from build123d import *

# Parameters (mm, degrees)
SKETCH1_W           = 42
SKETCH1_H           = 42
SKETCH1_R           = 1.7
SKETCH1_R_2         = 11.5
BOSS_EXTRUDE1_DEPTH = 4
SKETCH2_W           = 55
SKETCH2_H           = 80
SKETCH2_R           = 4.05
SKETCH2_W_2         = 36
SKETCH2_H_2         = 29
BOSS_EXTRUDE2_DEPTH = 10
BOSS_EXTRUDE4_DEPTH = 30.5
SKETCH5_W           = 42
SKETCH5_H           = 26.825
BOSS_EXTRUDE5_DEPTH = 42
SKETCH6_R           = 1.7
CUT_EXTRUDE1_DEPTH  = 83.547898974
SKETCH7_R           = 3.05
CUT_EXTRUDE2_DEPTH  = 56.825
SKETCH3_R           = 4.05
BOSS_EXTRUDE7_DEPTH = 3
SKETCH8_R           = 0.8
CUT_EXTRUDE3_DEPTH  = 1
BOSS_EXTRUDE8_DEPTH = 61.325
SKETCH10_R          = 2
CUT_EXTRUDE4_DEPTH  = 5
SKETCH11_R          = 2.25
CUT_EXTRUDE5_DEPTH  = 14
SKETCH12_W          = 8
SKETCH12_H          = 4
CUT_EXTRUDE6_DEPTH  = 13
CUT_EXTRUDE7_DEPTH  = 0.5


with BuildPart() as part:
    # Sketch1 → Boss-Extrude1 (new body)
    with BuildSketch(Plane(origin=(0, 0, 0), x_dir=(1, 0, 0), z_dir=(0, 1, 0))):
        with Locations((21, 21)):
            Rectangle(SKETCH1_W, SKETCH1_H)
        with Locations(Location((5.5, 36.5, 0), (0, 0, 270))):
            Circle(SKETCH1_R, mode=Mode.SUBTRACT)
        with Locations(Location((36.5, 36.5, 0), (0, 0, 270))):
            Circle(SKETCH1_R, mode=Mode.SUBTRACT)
        with Locations(Location((5.5, 5.5, 0), (0, 0, 270))):
            Circle(SKETCH1_R, mode=Mode.SUBTRACT)
        with Locations(Location((36.5, 5.5, 0), (0, 0, 270))):
            Circle(SKETCH1_R, mode=Mode.SUBTRACT)
        with Locations(Location((21, 21, 0), (0, 0, 270))):
            Circle(SKETCH1_R_2, mode=Mode.SUBTRACT)
    extrude(amount=BOSS_EXTRUDE1_DEPTH)

    # Sketch2 → Boss-Extrude2 (add)
    with BuildSketch(Plane.XY):
        with Locations((14.5, 21.325)):
            Rectangle(SKETCH2_W, SKETCH2_H)
        with Locations((2, 52.325)):
            Circle(SKETCH2_R, mode=Mode.SUBTRACT)
        with Locations((2, -9.675)):
            Circle(SKETCH2_R, mode=Mode.SUBTRACT)
        with Locations((18, 20)):
            Rectangle(SKETCH2_W_2, SKETCH2_H_2, mode=Mode.SUBTRACT)
    extrude(amount=BOSS_EXTRUDE2_DEPTH)

    # Sketch4 → Boss-Extrude4 (add)
    with BuildSketch(Plane(origin=(0, 4, 0), x_dir=(1, 0, 0), z_dir=(0, 1, 0))):
        with BuildLine():
            Line((0, 21), (9.5, 21))
            ThreePointArc((9.5, 21), (21, 32.5), (32.5, 21))
            Line((32.5, 21), (42, 21))
            Line((42, 21), (42, 42))
            Line((42, 42), (0, 42))
            Line((0, 42), (0, 21))
        make_face()
    extrude(amount=BOSS_EXTRUDE4_DEPTH)

    # Sketch5 → Boss-Extrude5 (add)
    with BuildSketch(Plane(origin=(0, 0, 0), x_dir=(-1, 0, 0), z_dir=(0, 0, -1))):
        with Locations((-21, 47.9125)):
            Rectangle(SKETCH5_W, SKETCH5_H)
    extrude(amount=BOSS_EXTRUDE5_DEPTH)

    # Sketch6 → Cut-Extrude1 (cut, through all)
    with BuildSketch(Plane.XZ.offset(-4)):
        with Locations(Location((5.5, -36.5, 0), (0, 0, 270))):
            Circle(SKETCH6_R)
        with Locations(Location((36.5, -36.5, 0), (0, 0, 270))):
            Circle(SKETCH6_R)
    extrude(amount=-CUT_EXTRUDE1_DEPTH, mode=Mode.SUBTRACT)

    # Sketch7 → Cut-Extrude2 (cut)
    with BuildSketch(Plane(origin=(0, 61.325, 0), x_dir=(1, 0, 0), z_dir=(0, 1, 0))):
        with Locations(Location((5.5, 36.5, 0), (0, 0, 180))):
            Circle(SKETCH7_R)
        with Locations(Location((36.5, 36.5, 0), (0, 0, 180))):
            Circle(SKETCH7_R)
        with Locations(Location((5.5, 5.5, 0), (0, 0, 180))):
            Circle(SKETCH7_R)
        with Locations(Location((36.5, 5.5, 0), (0, 0, 180))):
            Circle(SKETCH7_R)
    extrude(amount=-CUT_EXTRUDE2_DEPTH, mode=Mode.SUBTRACT)

    # Sketch3 → Boss-Extrude7 (add)
    with BuildSketch(Plane(origin=(0, 0, 0), x_dir=(-1, 0, 0), z_dir=(0, 0, -1))):
        with Locations((-2, -9.675)):
            Circle(SKETCH3_R)
        with Locations((-2, 52.325)):
            Circle(SKETCH3_R)
    extrude(amount=-BOSS_EXTRUDE7_DEPTH)

    # Sketch8 → Cut-Extrude3 (cut)
    with BuildSketch(Plane(origin=(0, 61.325, 0), x_dir=(1, 0, 0), z_dir=(0, 1, 0))):
        with Locations(Location((0.450490451, -5.1, 0), (0, 0, 180))):
            Circle(SKETCH8_R)
        with Locations(Location((7.148741473, -4.946920802, 0), (0, 0, 180))):
            Circle(SKETCH8_R)
    extrude(amount=-CUT_EXTRUDE3_DEPTH, mode=Mode.SUBTRACT)

    # Sketch9 → Boss-Extrude8 (add)
    with BuildSketch(Plane(origin=(0, 61.325, 0), x_dir=(1, 0, 0), z_dir=(0, 1, 0))):
        Polygon((-13, -10), (-19, -10), (-19, 60), (42, 60), (42, 42), (0, 42), (0, 0), (-13, 0), align=None)
    extrude(amount=-BOSS_EXTRUDE8_DEPTH)

    # Sketch10 → Cut-Extrude4 (cut)
    with BuildSketch(Plane.XZ):
        with Locations(Location((-6.5, -52.5, 0), (0, 0, 270))):
            Circle(SKETCH10_R)
        with Locations(Location((-6.5, -37.5, 0), (0, 0, 270))):
            Circle(SKETCH10_R)
    extrude(amount=-CUT_EXTRUDE4_DEPTH, mode=Mode.SUBTRACT)

    # Sketch11 → Cut-Extrude5 (cut)
    with BuildSketch(Plane(origin=(0, 0, -60), x_dir=(-1, 0, 0), z_dir=(0, 0, -1))):
        with Locations((-26, 53.325)):
            Circle(SKETCH11_R)
        with Locations((-11, 53.325)):
            Circle(SKETCH11_R)
    extrude(amount=-CUT_EXTRUDE5_DEPTH, mode=Mode.SUBTRACT)

    # Sketch12 → Cut-Extrude6 (cut)
    with BuildSketch(Plane(origin=(0, 61.325, 0), x_dir=(1, 0, 0), z_dir=(0, 1, 0))):
        with Locations((11, 51)):
            Rectangle(SKETCH12_W, SKETCH12_H)
        with Locations((26, 51)):
            Rectangle(SKETCH12_W, SKETCH12_H)
    extrude(amount=-CUT_EXTRUDE6_DEPTH, mode=Mode.SUBTRACT)

    # Sketch13 → Cut-Extrude7 (cut)
    with BuildSketch(Plane(origin=(42, 0, 0), x_dir=(0, 0, -1), z_dir=(1, 0, 0))):
        Polygon((40.371794872, 29.25), (35.756410256, 19.25), (36.731971154, 19.25), (38.210336538, 22.455128205), (42.743589744, 22.455128205), (44.264022436, 19.25), (45.243589744, 19.25), (40.5, 29.25), align=None)
        Polygon((40.445913462, 27.30088141), (42.256810897, 23.480769231), (38.683092949, 23.480769231), align=None, mode=Mode.SUBTRACT)
    extrude(amount=-CUT_EXTRUDE7_DEPTH, mode=Mode.SUBTRACT)


solid = part.part
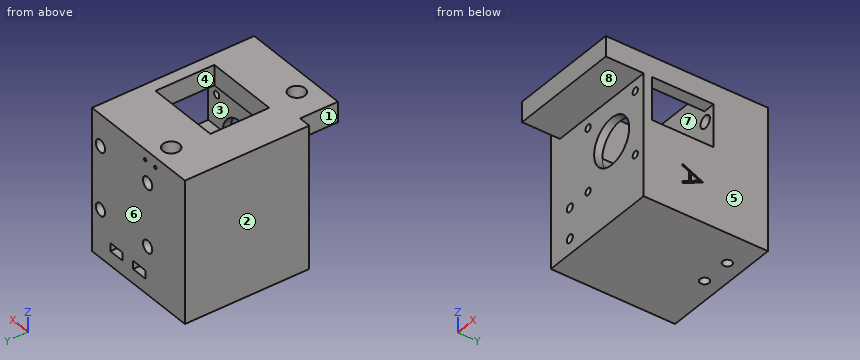
Design review of the part built by this model. Coordinates are the model's own, in mm. Face numbers are marked on the shaded views. A direction names the side the tool comes from. Give positions to 0.01 mm unless a question says otherwise; leave off trailing zeros. Loops run counter-clockwise (first coordinate to the right, second up) from the corner with the lowest first, then second, coordinate; pieces in that order, holes last. Notation, with made-up numbers: M 85,-4 L 124,-4 A36 cw 124,34 Z; hole C 64,65.5 d3. An arc over 180 degrees is marked long. Write item = value, one per line.
Q1. Draft analysis for pull direction Y (two halves, no side actions). For the marked faces 6, 7 and 8, state which applies: +Y half, -Y half, draft (parallel to the pull), parting line (faces both ways), or undercut.
Output values:
face_6 = +Y half
face_7 = undercut
face_8 = draft
Q2. To check wall thickness, follow line 1 (Y direction, x = 2, z = 4.75) (3 decimals); line 2 (Z direction, x = 36, y = 51); line 3 (Y direction, x = 6.5, z = -11.5) (3 decimals). State the ranges of each line that lie inside material, in increasing order. Write a range as [from, to].
Output values:
line_1 = [-18.675, -13.725], [-5.625, 5.5], [34.5, 48.275], [56.375, 61.325]
line_2 = [-60, -39.51], [-33.49, -8.51], [-2.49, 10]
line_3 = [0, 4], [34.5, 61.325]
Q3. For the marked faces 1, 2, 3, 4 and 5, list the 3-axis set-ups (+Z, -Z, +X, -X, +Y, -Y) from which the entire face can be reached by the end or side of a thin tool; tool diameter is ignored.
Output values:
face_1 = +Z, -Z, -X, -Y
face_2 = +Z, -Z, -X, +Y, -Y
face_3 = +X
face_4 = +Z
face_5 = +Z, -Z, +X, +Y, -Y
Q4. We need section B-B (x = 11). Give the boundary of the cut face in (y, z) (3 decimals).
Output values:
outline = M -18.675,0 L 0,0 L 0,-15.321 L 4,-15.321 L 4,0 L 5.5,0 L 5.5,10 L -18.675,10 Z; M 0,-60 L 51.075,-60 L 51.075,-53 L 48.325,-53 L 48.325,-49 L 51.075,-49 L 51.075,-46 L 55.575,-46 L 55.575,-49 L 61.325,-49 L 61.325,10 L 34.5,10 L 34.5,-26.679 L 0,-26.679 Z; M 55.575,-60 L 61.325,-60 L 61.325,-53 L 55.575,-53 Z
Q5. We need section A-A (y = 31.5). Give the boundary of the cut face in (x, z).
Output values:
outline = M -19,-60 L 42,-60 L 42,-21 L 32.5,-21 A11.5 cw 9.5,-21 L 0,-21 L 0,10 L -19,10 Z; M 36,0 L 42,0 L 42,10 L 36,10 Z; hole C 5.5,-36.5 d6.1; hole C 36.5,-36.5 d6.1
Q6. We need section C-C (x = -6.5). Give the boundary of the cut face in (y, z) (3 decimals), plus the area to 3 significant figures.
Output values:
outline = M -18.675,0 L 0,0 L 0,-35.5 L 5,-35.5 L 5,-39.5 L 0,-39.5 L 0,-50.5 L 5,-50.5 L 5,-54.5 L 0,-54.5 L 0,-60 L 61.325,-60 L 61.325,10 L -18.675,10 Z
area = 4,440 mm^2
Q7. We need section D-D (z = -30). Give the boundary of the cut face in (x, y) (3 decimals), plus the area to 3 significant figures.
Output values:
outline = M -19,0 L 13.841,0 L 13.841,34.5 L 28.159,34.5 L 28.159,0 L 42,0 L 42,61.325 L -19,61.325 Z
area = 3,250 mm^2
Q8. Insertion check: pin 1 (10 mm diameter, centred on x = 13, y = -8, fed in from -Z); pin 2 (5.5 mm diameter, centred on x = 5.5, z = -5.5, fed in from -Y); pin 3 (2 mm diameter, centred on x = 26, y = 53, fed in from -Z). Each pin has a flat end and moves straight along its axis. Give the tip position at first contact, or say it passes through.
Output values:
pin_1 = 0
pin_2 = 0
pin_3 = -46
